Check sheet for the modelled part. Datum: model origin and axes. Units: mm. A direction names the side the tool comes from. Round coordinates to 2 decimals unless told otherwise and drop trailing zeros. Write each loop counter-clockwise with the first axis right and the second up, starting at its lowest first coordinate (ties: lowest second). Pieces come first, ordered by that corner, then holes.
Item 1: Section check B-B, the plane z = -4.5. Record the cut outline in (x, y), plus the area to 3 significant figures.
Item 2: Depth check by flat-ended pin: pin 1 (12 mm diameter, centred on x = 9.5, z = -7, fed in from -Y); pin 2 (8.5 mm diameter, centred on x = 3.5, y = -2, fed in from +Z); pin 3 (11 mm diameter, centred on y = 1.5, z = 7.5, fed in from +X); pin 4 (10 mm diameter, centred on x = 11.5, z = 9.5, fed in from -Y). Enter the tip coordinate at first touch or a pass-through.
Item 3: Release check for a two-part mould opening along X. For faces 4 (the cylindrical face through (-14.307, -4.506, 4.147)), 5 (the flat face through (4.386, 7.456, 9.57)), 6 (the flat face through (0, 14, 9.5)) record: pulls with the +X half, pulls with the -X half, needs draft (parallel to the pull), parting line crosses it, or undercut.
Item 4: Section check A-A, the plane z = 11.25. Record the cut outline in (x, y), plus the area to 3 significant figures.
Item 5: Material ranges on line 1 along Y through (x, z) = (0, -6); line 2 along Y through (x, z) = (0, -1); line 3 along X through (y, z) = (-0.25, -11.25), recorded low to high.
Item 6: Set-up check for faces 1 (the flat face through (4, -4, 4.5)), 2 (the flat face through (0, 13.5, 2)), 3 (the flat face through (0, -14, 9.5)): record each of +Z, -Z, +X, -X, +Y, -Y from which the full face is reachable in a straight line by a thin tool's end or side.
from build123d import *

# Parameters (mm, degrees)
SKETCH_1_R               = 15
SKETCH_1_R_2             = 5.25
EXTRUDE_1_DEPTH          = 14.5
CUT_EXTRUDE_1_DEPTH      = 10
FILLET_2_R               = 8
CUT_EXTRUDE_2_DEPTH      = 26.695330315
CUT_EXTRUDE_2_DEPTH_BACK = 26.695330315
SKETCH_3_W               = 15
SKETCH_3_H               = 1.5


with BuildPart() as part:
    # 草图1 → 凸台-拉伸1 (new, symmetric)
    with BuildSketch(Plane.XY):
        with Locations(Location((0, 0, 0), (0, 0, 180))):
            Circle(SKETCH_1_R)
        with Locations(Location((0, 0, 0), (0, 0, 180))):
            Circle(SKETCH_1_R_2, mode=Mode.SUBTRACT)
    extrude(amount=EXTRUDE_1_DEPTH, both=True)

    # 草图2 → 切除-拉伸1 (cut)
    with BuildSketch(Plane.XY.offset(14.5)):
        Polygon((0, 9.988159657), (-8.65, 4.994079828), (-8.65, -4.994079828), (0, -9.988159657), (8.65, -4.994079828), (8.65, 4.994079828), align=None)
    extrude(amount=-CUT_EXTRUDE_1_DEPTH, mode=Mode.SUBTRACT)

    # 圆角2
    fillet_2_edges = [part.edges().sort_by_distance(p)[0] for p in [
        (15, 0, -14.5),
    ]]
    fillet(fillet_2_edges, radius=FILLET_2_R)

    # 草图3 → 切除-拉伸2 (cut, two sides: drawn at the far end of the back side and taken through both)
    with BuildSketch(Plane(origin=(0, 0, 0), x_dir=(0, 0, -1), z_dir=(1, 0, 0)).offset(-CUT_EXTRUDE_2_DEPTH_BACK)):
        with Locations((-2, 14.25)):
            Rectangle(SKETCH_3_W, SKETCH_3_H)
        with Locations((-2, -14.25)):
            Rectangle(SKETCH_3_W, SKETCH_3_H)
    extrude(amount=CUT_EXTRUDE_2_DEPTH + CUT_EXTRUDE_2_DEPTH_BACK, mode=Mode.SUBTRACT)


solid = part.part
Values found:
1. outline: (-6.54, -13.5) - (6.54, -13.5) arc R15 ccw to (6.54, 13.5) - (-6.54, 13.5) arc R15 ccw to start; hole circle Ø10.5 at (0, 0)
1. area: 594 mm2
2. pin 1: stops at y = -14.58
2. pin 2: stops at z = 4.5
2. pin 3: stops at x = 15
2. pin 4: stops at y = -13.52
3. face 4: parting line crosses it
3. face 5: undercut
3. face 6: needs draft
4. outline: circle Ø30 at (0, 0); hole (-8.65, -4.99) - (0, -9.99) - (8.65, -4.99) - (8.65, 4.99) - (0, 9.99) - (-8.65, 4.99) - close
4. area: 448 mm2
5. line 1: y = -15 to -5.25, 5.25 to 15
5. line 2: y = -13.5 to -5.25, 5.25 to 13.5
5. line 3: x = -13.43 to -5.24, 5.24 to 13.43
6. face 1: +Z
6. face 2: +X, -X, +Y
6. face 3: +X, -X, -Y
